Here's how the part is built. I have some questions about the finished solid (model axes, mm). A direction names the side the tool comes from. Give positions to 0.01 mm unless a question says otherwise; leave off trailing zeros. Loops run counter-clockwise (first coordinate to the right, second up) from the corner with the lowest first, then second, coordinate; pieces in that order, holes last.
Q1. For faces 1 (the face through (-30, 10, 1)), 2 (the face through (-1.216, 1.115, 0.986)), 3 (the face through (30, 10, 1)), which set-ups out of +Z, -Z, +X, -X, +Y, -Y let a thin tool reach every point of the face, with its end or its side?
Q2. I need wall thicknesses on line 1 (Y direction, x = 0, z = 0.5); line 2 (Y direction, x = -20, z = 1.8); line 3 (Y direction, x = -33, z = 0.25). Which ranges of each line are inside material? Lowest first, please.
Q3. If we section it at C-C (x = 0): Please give me the cut outline in (y, z).
Q4. We'd pull the mould along Y, two halves only. Please class faces 4 (the face through (40, 0, 1)), 5 (the face through (-1, -10, 1)), 6 (the face through (28.35, 0.07, 0.99)), 7 (the face through (13.01, 12.85, 1.01)): +Y half, -Y half, draft (parallel to the pull), parting line (faces both ways), or undercut.
Q5. If we section it at D-D (y = 35.5): Please give me the cut outline in (x, z), plus the area to 3 significant figures.
Q6. If we section it at A-A (x = -30): Please give me the cut outline in (y, z), plus the area to 3 significant figures.
Q7. If we section it at B-B (z = 1.4): Give the number of separate pieces and of enclosed holes in the cut face, plus the area to 3 significant figures.
Q8. Will these pins go through, and if not, where does the flat tip stop? P1, Ø1, axis at x = -26.5, z = 1, coming from the +Y side; P2, Ø0.6, axis at y = 41, z = 1, coming from the -X side.
from build123d import *

# Parameters (mm, degrees)
SKETCH_1_R      = 1.65
EXTRUDE_1_DEPTH = 2
FILLET_1_R      = 10


with BuildPart() as part:
    # 草图1 → 凸台-拉伸1 (new body)
    with BuildSketch(Plane.XY):
        Polygon((10, 10), (30, 10), (40, 10), (40, -10), (30, -10), (-30, -10), (-40, -10), (-40, 10), (-30, 10), (-10, 10), (-10, 50), (10, 50), align=None)
        Circle(SKETCH_1_R, mode=Mode.SUBTRACT)
        with Locations((-20, 0)):
            Circle(SKETCH_1_R, mode=Mode.SUBTRACT)
        with Locations((20, 0)):
            Circle(SKETCH_1_R, mode=Mode.SUBTRACT)
        with Locations((0, 20)):
            Circle(SKETCH_1_R, mode=Mode.SUBTRACT)
        with Locations((0, 30)):
            Circle(SKETCH_1_R, mode=Mode.SUBTRACT)
        with Locations((0, 40)):
            Circle(SKETCH_1_R, mode=Mode.SUBTRACT)
        with Locations((30, 0)):
            Circle(SKETCH_1_R, mode=Mode.SUBTRACT)
        with Locations((-30, 0)):
            Circle(SKETCH_1_R, mode=Mode.SUBTRACT)
    extrude(amount=EXTRUDE_1_DEPTH)

    # 圆角1
    fillet_1_edges = [part.edges().sort_by_distance(p)[0] for p in [
        (-10, 10, 1),
        (10, 10, 1),
    ]]
    fillet(fillet_1_edges, radius=FILLET_1_R)


solid = part.part
Check sheet entries:
1. face 1: +Z, -Z, -X, +Y
1. face 2: +Z, -Z
1. face 3: +Z, -Z, +X, +Y
2. line 1: y = -10 to -1.65, 1.65 to 18.35, 21.65 to 28.35, 31.65 to 38.35, 41.65 to 50
2. line 2: y = -10 to -1.65, 1.65 to 10
2. line 3: y = -10 to 10
3. outline: (-10, 0) - (-1.65, 0) - (-1.65, 2) - (-10, 2) - close; (1.65, 0) - (18.35, 0) - (18.35, 2) - (1.65, 2) - close; (21.65, 0) - (28.35, 0) - (28.35, 2) - (21.65, 2) - close; (31.65, 0) - (38.35, 0) - (38.35, 2) - (31.65, 2) - close; (41.65, 0) - (50, 0) - (50, 2) - (41.65, 2) - close
4. face 4: draft
4. face 5: -Y half
4. face 6: undercut
4. face 7: +Y half
5. outline: (-10, 0) - (10, 0) - (10, 2) - (-10, 2) - close
5. area: 40.0 mm2
6. outline: (-10, 0) - (-1.65, 0) - (-1.65, 2) - (-10, 2) - close; (1.65, 0) - (10, 0) - (10, 2) - (1.65, 2) - close
6. area: 33.4 mm2
7. separate pieces: 1
7. enclosed holes: 8
7. area: 2,370 mm2
8. P1: stops at y = 10
8. P2: stops at x = -10
